Geometry check sheet. Reference: drawing and pictorial views, mm from the part's lowest x, y, z. Give positions to 0.01 mm unless a question says otherwise; leave off trailing zeros. Order: outer loops, then holes, each group sorted by start corner. A loop starts at its lowest first (then second) coordinate and runs counter-clockwise, first axis right, second up.
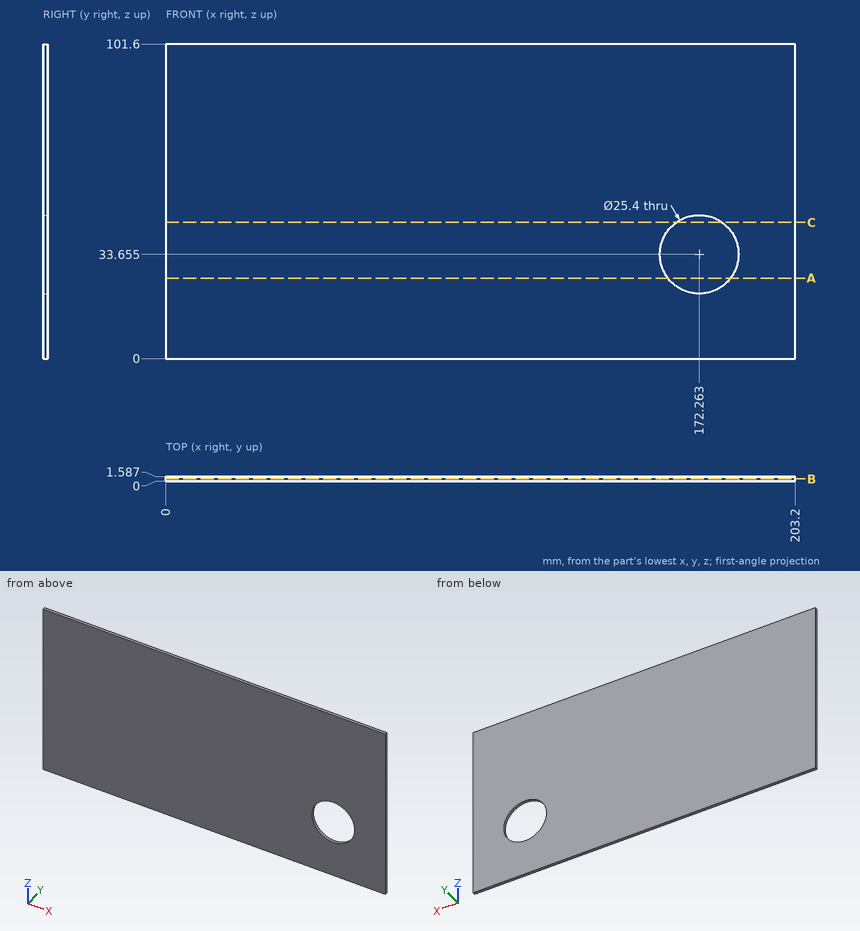
1) Section check C-C, the plane z = 44. Record the cut outline in (x, y) (1 decimal).
Recorded:
outline: (0, 0) - (164.9, 0) - (164.9, 1.6) - (0, 1.6) - close; (179.6, 0) - (203.2, 0) - (203.2, 1.6) - (179.6, 1.6) - close
2) Depth check by flat-ended pin: pin 1 Ø10 at (x, z) = (89, 73) entering from -Y. Enter the tip coordinate at first touch or a pass-through.
Recorded:
pin 1: stops at y = 0
3) Material ranges on L1, parallel to Z at x = 161.5, y = 0.5 (1 decimal); L2, parallel to X at y = 0.55, z = 43 (1 decimal); L3, parallel to Z at x = 183.5, y = 0.75 (1 decimal), recorded low to high.
Recorded:
L1: z = 0 to 26.9, 40.4 to 101.6
L2: x = 0 to 163.7, 180.9 to 203.2
L3: z = 0 to 27.7, 39.6 to 101.6
4) Section check A-A, the plane z = 26. Record the cut outline in (x, y).
Recorded:
outline: (0, 0) - (162.13, 0) - (162.13, 1.59) - (0, 1.59) - close; (182.4, 0) - (203.2, 0) - (203.2, 1.59) - (182.4, 1.59) - close
5) Section check B-B, the plane y = 0.85. Record the cut outline in (x, z) (1 decimal), then the cut area to 3 significant figures.
Recorded:
outline: (0, 0) - (203.2, 0) - (203.2, 101.6) - (0, 101.6) - close; hole circle Ø25.4 at (172.3, 33.7)
area: 20,100 mm2
